Can you work these out from the drawing? Everything is in mm from the part's minimum corner. Give positions to 0.01 mm unless a question says otherwise; leave off trailing zeros. Write each loop counter-clockwise with the first axis right and the second up, starting at its lowest first coordinate (ties: lowest second). Pieces come first, ordered by that corner, then holes. Notation, with made-up numbers: M 70,-26 L 106,-26 A25 cw 106,11 Z; hole C -1,-8.75 d9. An arc over 180 degrees is marked long. One line per item, written item: value.
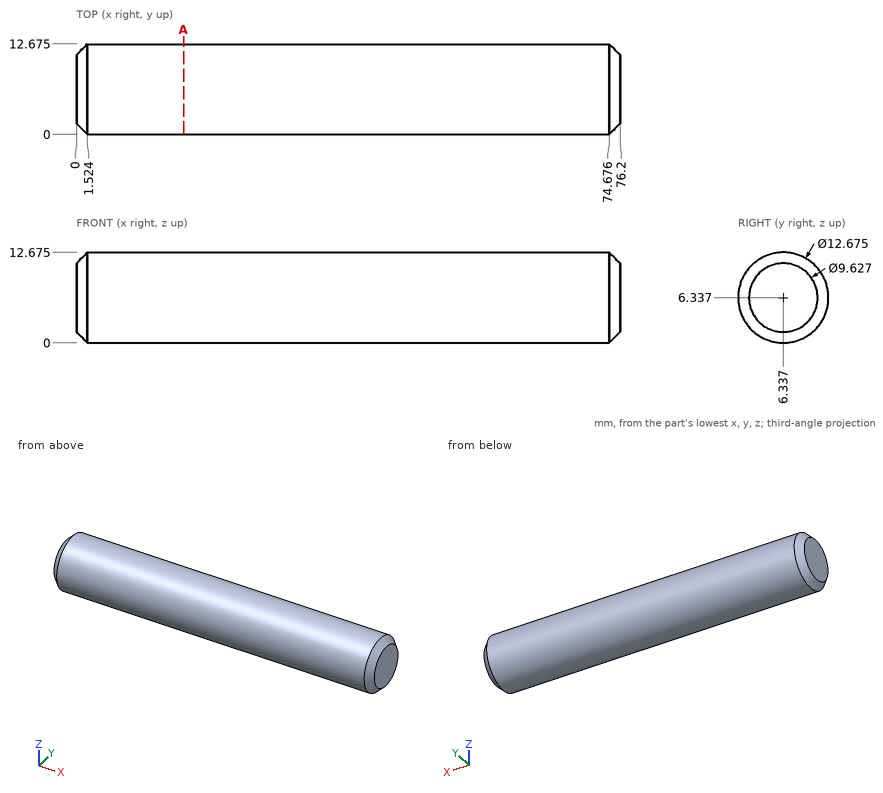
1) Please list where these lines run through material, in increasing order: L1, parallel to Y at x = 70.5, z = 10.25; L2, parallel to Y at x = 33, z = 6.75; L3, parallel to X at y = 3.25, z = 11.5. Write a range as from..to.
Outcome:
L1: y = 1.35..11.32
L2: y = 0.01..12.66
L3: x = 1.2..75
2) I'm going to push flat-ended pins straight in: pin 1 (6 mm diameter, centred on x = 12.5, y = 1.5, fed in from +Z); pin 2 (1 mm diameter, centred on x = 61.5, y = 8, fed in from -Z); pin 3 (1 mm diameter, centred on x = 17, y = 9.5, fed in from +Z). Where does each tip first touch, or does it pass through?
Outcome:
pin 1: stops at z = 12.4
pin 2: stops at z = 0.11
pin 3: stops at z = 12.09
3) If we section it at A-A, the plane x = 15: Write out the boundary of the cut face in (y, z) (1 decimal), then the cut area to 3 significant figures.
Outcome:
outline: C 6.3,6.3 d12.7
area: 126 mm^2
